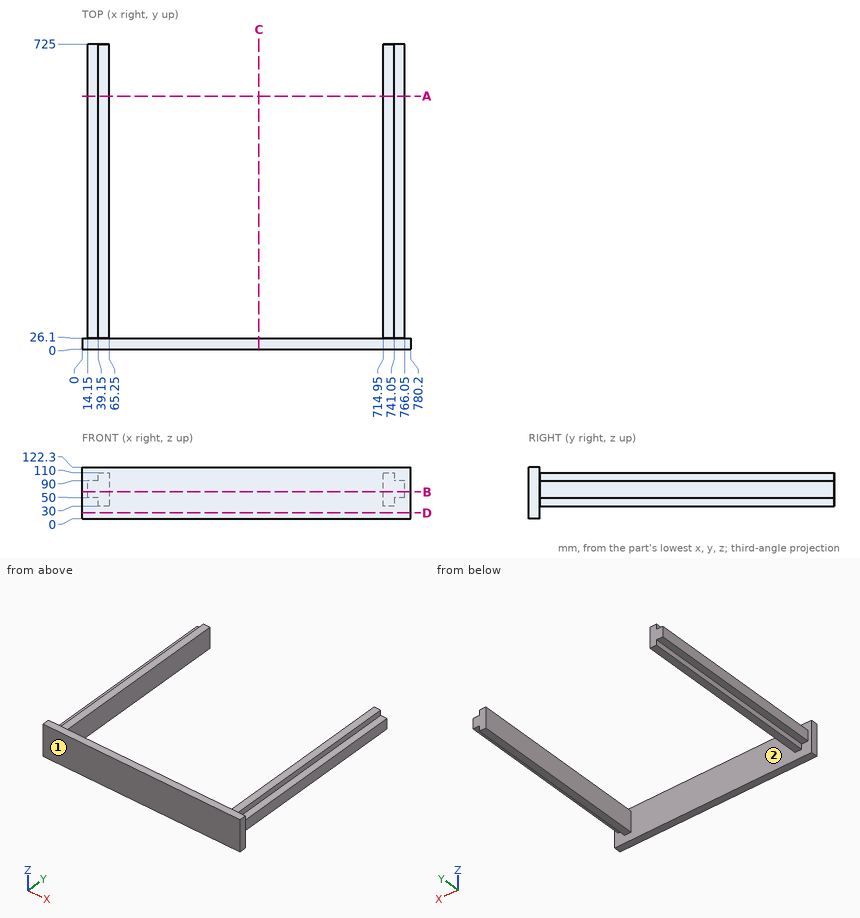
Study the drawing (mm; zero at the part's minimum x, y, z) and answer. Give positions to 0.01 mm unless a question says otherwise; leave off trailing zeros. Write each loop counter-clockwise with the first axis right and the second up, starting at its lowest first coordinate (ties: lowest second). Pieces come first, ordered by that corner, then holes. Notation, with made-up numbers: (33, -13) -> (79, -13) arc R27 cw to (79, 14) -> close; hole circle Ø4 at (66, -23.5). An arc over 180 degrees is marked (long way). Write item = value, one per line. Start each with the question number.
1) The part is cut by section B-B, the plane z = 64. Determine the outline of the cut face in (x, y).
2) The part is cut by section A-A, the plane y = 601. Determine the outline of the cut face in (x, z).
3) The part is cut by section D-D, the plane z = 14. Determine the outline of the cut face in (x, y), and give its area (3 significant figures).
4) Straight lines are drawn through the part: line 1 along X through (y, z) = (60.5, 89); line 2 along X through (y, z) = (127, 106); line 3 along Y through (x, z) = (629, 85). For each, find the intervals that lie inside material, in ascending order.
5) Each of these flat-tipped pins is pushed along its axis until it touches: pin 1 (3 mm diameter, centred on x = 272, z = 52.5, fed in from +Y); pin 2 (6 mm diameter, centred on y = 427, z = 96, fed in from -X); pin 3 (12 mm diameter, centred on y = 160.5, z = 76, fed in from +X). Where does it stop, or does it pass through?
6) The part is cut by section C-C, the plane x = 420. Determine the outline of the cut face in (y, z).
7) Determine the mould class of the marked faces 1 and 2 for opening direction X: +X half, -X half, draft (parallel to the pull), parting line (faces both ways), or undercut.
Solutions:
q1.outline = (0, 0) -> (780.2, 0) -> (780.2, 26.1) -> (766.05, 26.1) -> (766.05, 725) -> (714.95, 725) -> (714.95, 26.1) -> (65.25, 26.1) -> (65.25, 725) -> (14.15, 725) -> (14.15, 26.1) -> (0, 26.1) -> close
q2.outline = (14.15, 50) -> (39.15, 50) -> (39.15, 30) -> (65.25, 30) -> (65.25, 110) -> (39.15, 110) -> (39.15, 90) -> (14.15, 90) -> close; (714.95, 30) -> (741.05, 30) -> (741.05, 50) -> (766.05, 50) -> (766.05, 90) -> (741.05, 90) -> (741.05, 110) -> (714.95, 110) -> close
q3.outline = (0, 0) -> (780.2, 0) -> (780.2, 26.1) -> (0, 26.1) -> close
q3.area = 20,400 mm²
q4.line_1 = 14.15 to 65.25, 714.95 to 766.05
q4.line_2 = 39.15 to 65.25, 714.95 to 741.05
q4.line_3 = 0 to 26.1
q5.pin_1 = 26.1
q5.pin_2 = 39.15
q5.pin_3 = 766.05
q6.outline = (0, 0) -> (26.1, 0) -> (26.1, 122.3) -> (0, 122.3) -> close
q7.face_1 = draft
q7.face_2 = undercut
